Work out the finished part from the listing and answer in its coordinate system (mm). A direction names the side the tool comes from. Give positions to 0.01 mm unless a question says otherwise; leave off trailing zeros. Loops run counter-clockwise (first coordinate to the right, second up) from the corner with the lowest first, then second, coordinate; pieces in that order, holes last.
from build123d import *

# Parameters (mm, degrees)
F1_W     = 41.275
F1_H     = 89.1649350524
F1_H_2   = 37.8350649476
F2_DEPTH = 41.275
F4_DEPTH = 41.275


# Not quite as in the source:
# - a variable given as a bare number and used for a length is read in inches; the dataset says mm whatever the document's units were


with BuildPart() as f2:
    # F1 (on Front) → F2 (new body, symmetric)
    with BuildSketch(Plane.XZ):
        with Locations((20.6375, -44.5824675262)):
            Rectangle(F1_W, F1_H)
        with Locations((-20.6375, -108.0824675262)):
            Rectangle(F1_W, F1_H_2)
        with Locations((20.6375, -108.0824675262)):
            Rectangle(F1_W, F1_H_2)
    extrude(amount=F2_DEPTH, both=True)

    # F1 (on Front) → F3 (revolve, intersect)
    with BuildSketch(Plane.XZ):
        with BuildLine():
            Line((41.275, -127), (0, -127))
            Line((0, -127), (0, -723.9))
            Line((0, -723.9), (22.225, -723.9))
            Line((22.225, -723.9), (38.1, -177.8))
            ThreePointArc((38.1, -177.8), (36.5217864477, -170.6516067761), (31.75, -165.1))
            Line((31.75, -165.1), (31.75, -139.7))
            ThreePointArc((31.75, -139.7), (35.2305301109, -136.3908180665), (36.5125, -131.7625))
            ThreePointArc((36.5125, -131.7625), (38.9267731534, -129.4142731534), (41.275, -127))
        make_face()
        with Locations((20.6375, -108.0824675262)):
            Rectangle(F1_W, F1_H_2)
        with BuildLine():
            Line((41.275, -89.1649350524), (41.275, -127))
            ThreePointArc((41.275, -127), (55.2047536515, -109.2185398369), (65.6004882321, -89.1649350524))
            Line((65.6004882321, -89.1649350524), (41.275, -89.1649350524))
        make_face()
    revolve(axis=Axis((0, 0, -361.95), (0, 0, -1)), mode=Mode.INTERSECT)

    # F1 (on Front) → F4 (join, symmetric)
    with BuildSketch(Plane.XZ):
        with Locations((-20.6375, -44.5824675262)):
            Rectangle(F1_W, F1_H)
        with Locations((20.6375, -44.5824675262)):
            Rectangle(F1_W, F1_H)
    extrude(amount=F4_DEPTH, both=True)

    # F1 (on Front) → F5 (revolve)
    with BuildSketch(Plane.XZ):
        with BuildLine():
            Line((41.275, -127), (0, -127))
            Line((0, -127), (0, -723.9))
            Line((0, -723.9), (22.225, -723.9))
            Line((22.225, -723.9), (38.1, -177.8))
            ThreePointArc((38.1, -177.8), (36.5217864477, -170.6516067761), (31.75, -165.1))
            Line((31.75, -165.1), (31.75, -139.7))
            ThreePointArc((31.75, -139.7), (35.2305301109, -136.3908180665), (36.5125, -131.7625))
            ThreePointArc((36.5125, -131.7625), (38.9267731534, -129.4142731534), (41.275, -127))
        make_face()
    revolve(axis=Axis((0, 0, -361.95), (0, 0, -1)))


solid = f2.part
Item 1: For faces 1 (the face through (-24.024, 18.421, -447.027)), 2 (the face through (-1, -41.275, -63)), determine the directions among +Z, -Z, +X, -X, +Y, -Y from which every point of the face is accessible in a straight line to the end or side of a thin tool.
Item 2: Find section A-A, the plane z = -453. Write down the section's boundary in (x, y), plus the area to 3 significant figures.
Item 3: Determine the mould class of faces 3 (the face through (-6.883, 30.995, -152.222)), 4 (the face through (41.275, -1, -64)), 5 (the face through (1, -1, 0)) for opening direction Z: released by +Z, released by -Z, zero draft, split by the parting line, or undercut.
Item 4: Consider line 1 (Y direction, x = 21, z = -670.5); line 2 (X direction, y = 17.5, z = -633); line 3 (Z direction, x = -38, y = 35). Determine where each line is inside the solid, lowest interval first.
Item 5: Flat-ended cylindrical pins translate along their axes: pin 1 Ø3 at (x, z) = (8, -311.5) entering from -Y; pin 2 Ø6 at (y, z) = (4.5, -148) entering from +X; pin 3 Ø8 at (x, y) = (-1.5, -26) entering from +Z; pin 4 Ø8 at (x, z) = (23, -394.5) entering from +Y. Find the tip coordinate at first contact, or state that the pin passes through.
Ans:
1. face 1: -Z
1. face 2: +Z, -Z, +X, -X, -Y
2. outline: circle Ø60.2 at (0, 0)
2. area: 2,850 mm2
3. face 3: undercut
3. face 4: zero draft
3. face 5: released by +Z
4. line 1: y = -11.15 to 11.15
4. line 2: x = -17.67 to 17.67
4. line 3: z = -114.43 to 0
5. pin 1: stops at y = -33.59
5. pin 2: stops at x = 31.71
5. pin 3: stops at z = 0
5. pin 4: stops at y = 25.5
